from build123d import *

# Parameters (mm, degrees)
SKETCH1_W           = 25.4
SKETCH1_H           = 25.4
SKETCH1_W_2         = 20.32
SKETCH1_H_2         = 20.32
BOSS_EXTRUDE1_DEPTH = 190.5
CUT_EXTRUDE1_DEPTH  = 193.605036279
SKETCH3_R           = 3.175
CUT_EXTRUDE2_DEPTH  = 193.605036279
SKETCH4_R           = 2.38125
CUT_EXTRUDE3_DEPTH  = 193.605036279


with BuildPart() as part:
    # Sketch1 → Boss-Extrude1 (new body)
    with BuildSketch(Plane(origin=(0, 0, 0), x_dir=(0, 0, -1), z_dir=(1, 0, 0))):
        Rectangle(SKETCH1_W, SKETCH1_H)
        Rectangle(SKETCH1_W_2, SKETCH1_H_2, mode=Mode.SUBTRACT)
    extrude(amount=BOSS_EXTRUDE1_DEPTH)

    # Sketch2 → Cut-Extrude1 (cut, through all)
    with BuildSketch(Plane.XY.offset(12.7)):
        Polygon((0, -12.7), (25.4, 12.7), (0, 12.7), align=None)
    extrude(amount=-CUT_EXTRUDE1_DEPTH, mode=Mode.SUBTRACT)

    # Sketch3 → Cut-Extrude2 (cut, through all)
    with BuildSketch(Plane(origin=(0, 12.7, 0), x_dir=(1, 0, 0), z_dir=(0, 1, 0))):
        with Locations(Location((177.8, 0, 0), (0, 0, 270))):
            Circle(SKETCH3_R)
        with Locations(Location((39.37, 0, 0), (0, 0, 270))):
            Circle(SKETCH3_R)
    extrude(amount=-CUT_EXTRUDE2_DEPTH, mode=Mode.SUBTRACT)

    # Sketch4 → Cut-Extrude3 (cut, through all)
    with BuildSketch(Plane.XY.offset(12.7)):
        with Locations((95.25, 0)):
            Circle(SKETCH4_R)
        with Locations((120.65, 0)):
            Circle(SKETCH4_R)
        with Locations((69.85, 0)):
            Circle(SKETCH4_R)
    extrude(amount=-CUT_EXTRUDE3_DEPTH, mode=Mode.SUBTRACT)


solid = part.part
Here's how the part is built. I have some questions about the finished solid (model axes, mm). A direction names the side the tool comes from. Round coordinates to 2 decimals unless told otherwise and drop trailing zeros. Loops run counter-clockwise (first coordinate to the right, second up) from the corner with the lowest first, then second, coordinate; pieces in that order, holes last. Notation, with made-up numbers: (-8, 52.5) - (17, 52.5) arc R10 ccw to (17, 69.5) - close; hole circle Ø11 at (55.25, 54). An arc over 180 degrees is marked (long way). One line per question, with ' | ' between items. Start each with the question number.
Q1. Please list where these lines run through material, in increasing order: line 1 (Y direction, x = 174, z = 0.75); line 2 (X direction, y = 10.95, z = 0) (3 decimals). Write a range as [from, to].
Q2. I want a section at C-C (x = 177.8). Write out the boundary of the cut face in (y, z) (3 decimals).
Q3. Will these pins go through, and if not, where does the flat tip stop? pin 1 (5 mm diameter, centred on y = -7.5, z = -6, fed in from -X); pin 2 (6 mm diameter, centred on y = 7.5, z = 3, fed in from -X).
Q4. I want a section at D-D (z = 0). Write out the boundary of the cut face in (x, y) (3 decimals), then the cut area to 3 significant figures.
Q5. We'd pull the mould along X, two halves only. Please class faces 3 (the flat face through (94, -3, -12.7)), 4 (the cylindrical face through (180.95, -11.41, -0.41)), 5 (the flat face through (12.5, -0.2, -11.1)), 6 (the cylindrical face through (92.87, 0.1, 11.45)): +X half, -X half, draft (parallel to the pull), parting line (faces both ways), or undercut.
Q6. I want a section at A-A (z = -7.25). Write out the boundary of the cut face in (x, y).
Q7. For faces 1 (the flat face through (106, 10.16, 0)), 2 (the cylindrical face through (92.87, 0.1, -11.41)), which set-ups out of +Z, -Z, +X, -X, +Y, -Y let a thin tool reach every point of the face, with its end or its side?
Q8. I want a section at B-B (y = 0). State how many separate pieces and enclosed holes the cut face has, then the cut area to 3 significant figures.
Response values:
1) line 1: y = [-12.7, -10.16], [10.16, 12.7] | line 2: x = [23.65, 36.195], [42.545, 174.625], [180.975, 190.5]
2) outline: (-12.7, -12.7) - (12.7, -12.7) - (12.7, -3.175) - (10.16, -3.175) - (10.16, -10.16) - (-10.16, -10.16) - (-10.16, -3.175) - (-12.7, -3.175) - close; (-12.7, 3.175) - (-10.16, 3.175) - (-10.16, 10.16) - (10.16, 10.16) - (10.16, 3.175) - (12.7, 3.175) - (12.7, 12.7) - (-12.7, 12.7) - close
3) pin 1: passes through | pin 2: stops at x = 22.86
4) outline: (0, -12.7) - (36.195, -12.7) - (36.195, -10.16) - (2.54, -10.16) - close; (22.86, 10.16) - (36.195, 10.16) - (36.195, 12.7) - (25.4, 12.7) - close; (42.545, -12.7) - (174.625, -12.7) - (174.625, -10.16) - (42.545, -10.16) - close; (42.545, 10.16) - (174.625, 10.16) - (174.625, 12.7) - (42.545, 12.7) - close; (180.975, -12.7) - (190.5, -12.7) - (190.5, -10.16) - (180.975, -10.16) - close; (180.975, 10.16) - (190.5, 10.16) - (190.5, 12.7) - (180.975, 12.7) - close | area: 839 mm²
5) face 3: draft | face 4: undercut | face 5: -X half | face 6: undercut
6) outline: (0, -12.7) - (190.5, -12.7) - (190.5, -10.16) - (2.54, -10.16) - close; (22.86, 10.16) - (190.5, 10.16) - (190.5, 12.7) - (25.4, 12.7) - close
7) face 1: +X, -X | face 2: +Z, -Z
8) separate pieces: 8 | enclosed holes: 0 | area: 831 mm²
